Answer from the drawing. Dimensions are ordinates in mm from the lowest x, y and z of the part. Round coordinates to 2 decimals unless told otherwise and drop trailing zeros. Loops run counter-clockwise (first coordinate to the right, second up) from the corner with the lowest first, then second, coordinate; pieces in that order, holes last. Notation, with made-up numbers: M 43.25,-33 L 60.25,-33 A12 cw 60.25,-19 Z; hole C 89.5,83.5 d9. An arc over 180 degrees is marked long. Answer as a JSON object with one key per item and string values.
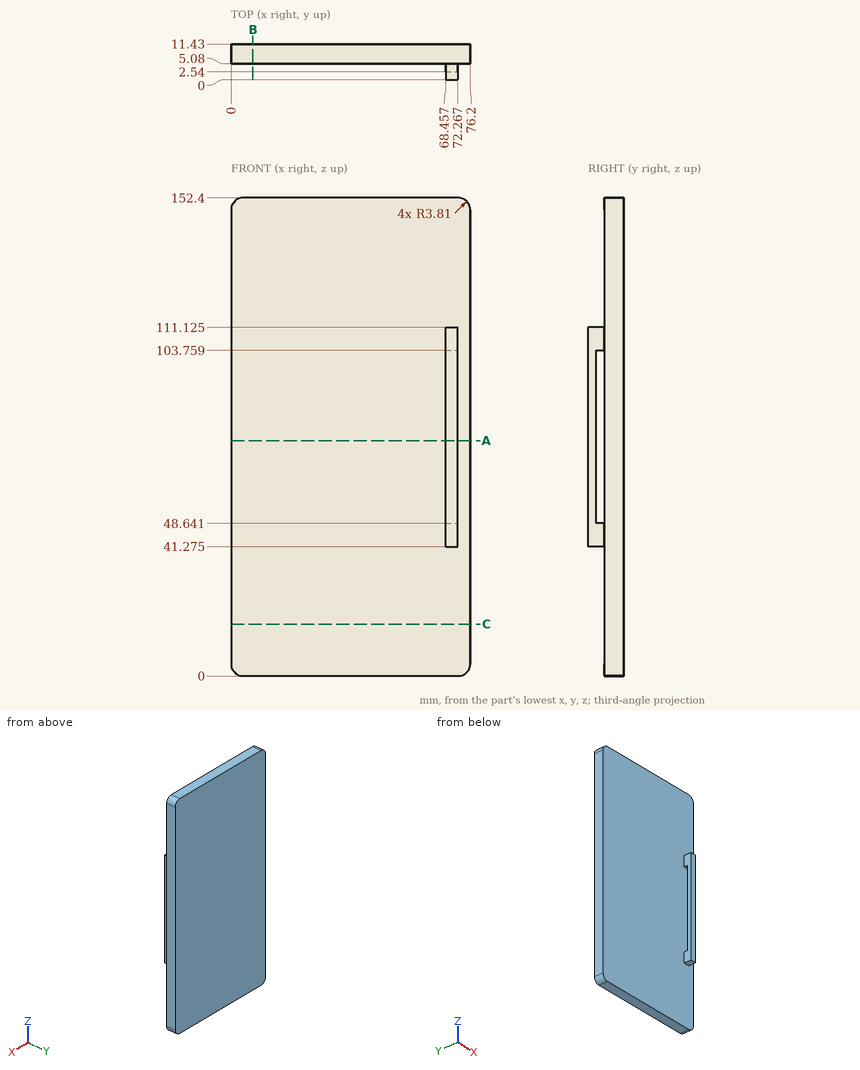
Item 1: The part is cut by section B-B (x = 7). Give the vertices of the cut face in (y, z).
Values follow:
{"outline": "M 5.08,0 L 11.43,0 L 11.43,152.4 L 5.08,152.4 Z"}
Item 2: The part is cut by section A-A (z = 75). Give the vertices of the cut face in (x, y).
Values follow:
{"outline": "M 0,5.08 L 76.2,5.08 L 76.2,11.43 L 0,11.43 Z; M 68.46,0 L 72.27,0 L 72.27,2.54 L 68.46,2.54 Z"}
Item 3: Flat-ended cylindrical pins translate along their axes: P1, Ø2.5, axis at y = 1.5, z = 87, coming from the -X side; P2, Ø2, axis at x = 70, y = 3, coming from the +Z side (3 decimals); P3, Ø23, axis at x = 43, z = 44, coming from the -Y side; P4, Ø3, axis at x = 56.5, y = 2, coming from the -Z side. Find the tip coordinate at first contact, or state that the pin passes through.
Values follow:
{"P1": "x = 68.46", "P2": "z = 111.125", "P3": "y = 5.08", "P4": "through"}
Item 4: Straight lines are drawn through the part: line 1 (Y direction, x = 25, z = 69); line 2 (X direction, y = 0.5, z = 48). For each, find the intervals that lie inside material, in ascending order.
Values follow:
{"line 1": "5.08 to 11.43", "line 2": "68.46 to 72.27"}
Item 5: The part is cut by section C-C (z = 16.5). Give the vertices of the cut face in (x, y), then the cut area to 3 significant figures.
Values follow:
{"outline": "M 0,5.08 L 76.2,5.08 L 76.2,11.43 L 0,11.43 Z", "area": "484 mm^2"}
